The model under review builds one solid part; all positions refer to its coordinate system, in mm. Give positions to 0.01 mm unless a question says otherwise; leave off trailing zeros. Order: outer loops, then holes, each group sorted by start corner. A loop starts at its lowest first (then second) coordinate and runs counter-clockwise, first axis right, second up. Notation, with made-up numbers: (38, 63) - (68, 63) arc R25 cw to (68, 86) - close; hole circle Ø9 at (36, -29). An arc over 180 degrees is marked (long way). Use CSV: the item, a comma, the result in double quotes. Start each with the question number.
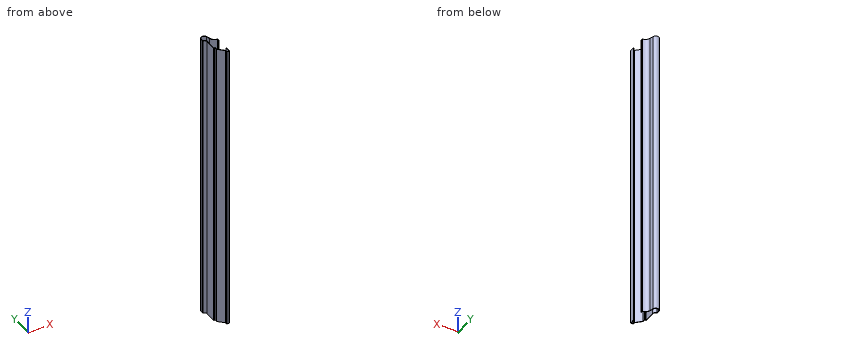
```python
from build123d import *

# Parameters (mm, degrees)
EXTRUDE_THIN1_DEPTH = 666.75
FILLET1_R           = 0.889


with BuildPart() as part:
    # Sketch1 → Extrude-Thin1 (new body)
    with BuildSketch(Plane.XY):
        with BuildLine():
            Line((0, 11.1125), (0, 0))
            Line((0, 0), (-6.35, 0))
            Line((-6.35, 0), (-6.35, 4.7625))
            Line((-6.35, 4.7625), (-19.05, 17.4625))
            Line((-19.05, 17.4625), (-19.05, 22.621875))
            Line((-19.05, 22.621875), (-22.225, 22.225))
            Line((-22.225, 22.225), (-22.225, 47.681988686))
            ThreePointArc((-22.225, 47.681988686), (-24.143830542, 51.882118892), (-28.575, 53.18125))
            Line((-28.575, 53.18125), (-28.575, 59.53125))
            ThreePointArc((-28.575, 59.53125), (-22.468372416, 66.599314881), (-14.588636772, 61.583519054))
            Line((-14.588636772, 61.583519054), (-12.164645739, 53.501521681))
            ThreePointArc((-12.164645739, 53.501521681), (-7.581369446, 46.96114151), (0, 44.45))
            Line((0, 44.45), (0, 39.6875))
            Line((0, 39.6875), (-0.889, 39.6875))
            Line((-0.889, 39.6875), (-0.889, 43.59011062))
            ThreePointArc((-0.889, 43.59011062), (-8.464520872, 46.519251795), (-13.016170941, 53.246128199))
            Line((-13.016170941, 53.246128199), (-15.440161973, 61.328125572))
            ThreePointArc((-15.440161973, 61.328125572), (-22.339308293, 65.719733473), (-27.686, 59.53125))
            Line((-27.686, 59.53125), (-27.686, 54.12653483))
            ThreePointArc((-27.686, 54.12653483), (-23.190217566, 52.20566736), (-21.336, 47.681988686))
            Line((-21.336, 47.681988686), (-21.336, 23.232043392))
            Line((-21.336, 23.232043392), (-18.161, 23.628918392))
            Line((-18.161, 23.628918392), (-18.161, 17.830735857))
            Line((-18.161, 17.830735857), (-5.461, 5.130735857))
            Line((-5.461, 5.130735857), (-5.461, 0.889))
            Line((-5.461, 0.889), (-0.889, 0.889))
            Line((-0.889, 0.889), (-0.889, 11.1125))
            Line((-0.889, 11.1125), (0, 11.1125))
        make_face()
    extrude(amount=-EXTRUDE_THIN1_DEPTH)

    # Fillet1
    fillet1_edges = [part.edges().sort_by_distance(p)[0] for p in [
        (-18.161, 23.628918392, -333.375),
        (-5.461, 5.130735857, -333.375),
        (0, 0, -333.375),
        (-6.35, 0, -333.375),
        (-19.05, 17.4625, -333.375),
        (-22.225, 22.225, -333.375),
        (-28.575, 53.18125, -333.375),
        (0, 44.45, -333.375),
    ]]
    fillet(fillet1_edges, radius=FILLET1_R)


solid = part.part
```
1. Clearance check with flat-ended pins moving along their axes: pin 1 (1 mm diameter, centred on x = -0.5, z = -290, fed in from -Y); pin 2 (8 mm diameter, centred on x = -25.5, z = -334, fed in from -Y); pin 3 (2.5 mm diameter, centred on y = 19.5, z = -427, fed in from +X); pin 4 (8 mm diameter, centred on x = -6, z = -115, fed in from +Y). State where each tip first meets the part, or that it passes through.
2. To check wall thickness, follow L1, parallel to X at y = 42, z = -192.5 (3 decimals); L2, parallel to X at y = 19.5, z = -510; L3, parallel to X at y = 53.5, z = -535. State the ranges of each line that lie inside material, in increasing order. Write a range as [from, to].
3. Consider section A-A (y = 33). Give the boundary of the cut face in (x, z) (3 decimals), and give its area (3 significant figures).
Answers follow:
1,pin 1,"stops at y = 0"
1,pin 2,"stops at y = 22.36"
1,pin 3,"stops at x = -18.16"
1,pin 4,"stops at y = 49.32"
2,L1,"x = [-22.225, -21.336], [-0.889, 0]"
2,L2,"x = [-19.05, -18.16]"
2,L3,"x = [-28.32, -25.01], [-13.09, -12.16]"
3,outline,"(-22.225, -666.75) - (-21.336, -666.75) - (-21.336, 0) - (-22.225, 0) - close"
3,area,"593 mm^2"
